Here's how the part is built. I have some questions about the finished solid (model axes, mm). A direction names the side the tool comes from. Give positions to 0.01 mm unless a question says otherwise; leave off trailing zeros. Loops run counter-clockwise (first coordinate to the right, second up) from the corner with the lowest first, then second, coordinate; pieces in that order, holes last. Notation, with made-up numbers: (-1, 70.25) - (24, 70.25) arc R20 ccw to (24, 104.25) - close; hole circle Ø4 at (58.25, 55.25). An arc over 180 degrees is marked (long way). One line per item, written item: value. Start each with the question number.
Autodesk Inventor part; units mm, degrees
ref_plane "YZ Plane" through (0, 0, 0) normal (1, 0, 0) x (0, 1, 0)
ref_plane "XZ Plane" through (0, 0, 0) normal (0, 1, 0) x (-1, 0, 0)
ref_plane "XY Plane" through (0, 0, 0) normal (0, 0, 1) x (1, 0, 0)
sketch "Sketch1" plane through (0, 0, 0) normal (0, 1, 0) x (-1, 0, 0)
  circle A0 centre (0, 0) radius 1.65
  arc A1 (3.65, 0) -> (-3.65, 0) centre (0, 0) ccw
  line L0 (-3.65, 0) -> (-3.65, -11.35)
  line L1 (-3.65, -11.35) -> (3.65, -11.35)
  line L2 (3.65, -11.35) -> (3.65, 0)
  line L3 (0, 0) -> (0, -26.2529)
  line L4 (2.85, -11.35) -> (-2.85, -11.35)
  line L5 (-2.85, -9.35) -> (-2.85, -6.35)
  line L6 (-2.85, -6.35) -> (2.85, -6.35)
  line L7 (2.85, -6.35) -> (2.85, -9.35)
  line L8 (2.85, -9.35) -> (-2.85, -9.35)
  dimension "d0" = 3.3
  dimension "d1" = 2
  dimension "d2" = 15
  dimension "d3" = 5.7
  dimension "d4" = 5
  dimension "d5" = 2
  dimension "d13" = 3.65
  dimension "d14" = 7.3
  dimension "d15" = 0.8
extrude "Extrusion1" add sketch "Sketch1" along normal mid plane 3.5
sketch "Sketch3" plane through (0, 0, 0) normal (0, 1, 0) x (-1, 0, 0)
  line L0 (-2.85, -6.35) -> (2.85, -6.35) construction
  line L1 (2.85, -6.35) -> (2.85, -9.35) construction
  line L2 (2.85, -9.35) -> (-2.85, -9.35) construction
  line L3 (-2.85, -9.35) -> (-2.85, -6.35) construction
  circle A0 centre (0, 0) radius 1.65 construction
  arc A1 (3.65, 0) -> (-3.65, 0) centre (0, 0) ccw construction
  line L4 (-3.65, 0) -> (-3.65, -11.35)
  line L5 (-3.65, -11.35) -> (3.65, -11.35)
  line L6 (3.65, -11.35) -> (3.65, 0)
  line L7 (3.65, -11.35) -> (-3.65, -11.35)
  line L8 (-3.65, -11.35) -> (-3.65, -8.85)
  line L9 (-3.65, -8.85) -> (3.65, -8.85)
  line L10 (3.65, -8.85) -> (3.65, -11.35)
  line L11 (4.85, -4.85) -> (2.85, -4.85)
  line L12 (2.85, -4.85) -> (2.85, -11.35)
  line L13 (2.85, -11.35) -> (4.85, -11.35)
  line L14 (4.85, -11.35) -> (4.85, -4.85)
  line L15 (-2.85, -4.85) -> (-4.85, -4.85)
  line L16 (-4.85, -4.85) -> (-4.85, -11.35)
  line L17 (-4.85, -11.35) -> (-2.85, -11.35)
  line L18 (-2.85, -11.35) -> (-2.85, -4.85)
  line L19 (-2.85, -9.35) -> (-2.85, -6.35)
  line L20 (2.85, -6.35) -> (2.85, -9.35)
  dimension "d16" = 2
  dimension "d17" = 1.5
extrude "Extrusion2" add sketch "Sketch3" along normal mid plane 6
sketch "Sketch5" plane through (4.85, 3, -11.35) normal (0, 0, -1) x (-1, 0, 0)
  circle A0 centre (4.85, -3) radius 1.6
  dimension "d18" = 3.2
extrude "Extrusion4" cut sketch "Sketch5" against normal up to surface (2.5 mm away)
properties part number "connectiong-rod-star-side"
(1) Will these pins go through, and if not, where does the flat tip stop? pin 1 (4 mm diameter, centred on x = 1, z = -1, fed in from -Y); pin 2 (1.9 mm diameter, centred on x = 0, y = 0, fed in from -Z); pin 3 (1 mm diameter, centred on x = -3.5, y = 0, fed in from +Z).
(2) Please list where these lines run through material, in increasing order: probe 1 along Z at (x, y) = (0, 0.9); probe 2 along X at (y, z) = (1.8, -7); probe 3 along Y at (x, z) = (0.5, -2). Write a range as from..to.
(3) If we section it at A-A on x = 0: List the corners of the cut face in (y, z) for me.
(4) If we section it at C-C on y = 2.1: List the corners of the cut face in (x, z) for me, plus the area to 4 significant figures.
(5) If we mould it in two halves opening along X, with no side actions, what happens to faces 1 (the face through (-4, 0, -4.85)), 2 (the face through (3.65, 0, -2)), 3 (the face through (1.3, 1.3, -8.85))? For each: pulls with the +X half, pulls with the -X half, needs draft (parallel to the pull), parting line crosses it, or undercut.
(6) If we section it at B-B on z = -9.75: List the corners of the cut face in (x, y) for me, plus the area to 3 significant figures.
(7) If we section it at D-D on z = -7.25: List the corners of the cut face in (x, y) for me, plus the area to 3 significant figures.
(8) For faces 4 (the face through (1.27, -0.97, -10.12)), 5 (the face through (-3.65, 0, -2)), 6 (the face through (0, 3, -9)), 7 (the face through (-4.85, 0, -8)), 8 (the face through (0, 0, -6.35)), which set-ups out of +Z, -Z, +X, -X, +Y, -Y let a thin tool reach every point of the face, with its end or its side?
Found:
1. pin 1: y = -1.75
1. pin 2: z = -6.35
1. pin 3: z = 2.08
2. probe 1: -6.35..-1.65, 1.65..3.65
2. probe 2: -4.85..-2.85, 2.85..4.85
2. probe 3: -1.75..1.75
3. outline: (-3, -11.35) - (-1.6, -11.35) - (-1.6, -8.85) - (-3, -8.85) - close; (-1.75, -6.35) - (1.75, -6.35) - (1.75, -1.65) - (-1.75, -1.65) - close; (-1.75, 1.65) - (1.75, 1.65) - (1.75, 3.65) - (-1.75, 3.65) - close; (1.6, -11.35) - (3, -11.35) - (3, -8.85) - (1.6, -8.85) - close
4. outline: (-4.85, -11.35) - (4.85, -11.35) - (4.85, -4.85) - (2.85, -4.85) - (2.85, -8.85) - (-2.85, -8.85) - (-2.85, -4.85) - (-4.85, -4.85) - close
4. area: 40.25 mm^2
5. face 1: needs draft
5. face 2: pulls with the +X half
5. face 3: undercut
6. outline: (-4.85, -3) - (4.85, -3) - (4.85, 3) - (-4.85, 3) - close; hole circle Ø3.2 at (0, 0)
6. area: 50.2 mm^2
7. outline: (-4.85, -3) - (-2.85, -3) - (-2.85, 3) - (-4.85, 3) - close; (2.85, -3) - (4.85, -3) - (4.85, 3) - (2.85, 3) - close
7. area: 24.0 mm^2
8. face 4: -Z
8. face 5: +Z, -X, +Y, -Y
8. face 6: +Z, -Z, +X, -X, +Y
8. face 7: +Z, -Z, -X, +Y, -Y
8. face 8: +Y, -Y
